```python
from build123d import *

# Parameters (mm, degrees)
SKETCH1_W                 = 20
SKETCH1_H                 = 101.6
BASE_FLANGE1_DEPTH        = 0.7366
EDGE_FLANGE1_DEPTH        = 40.191036667
EDGE_FLANGE1_START        = 0.7366
EDGE_FLANGE1_FLAT_DEPTH   = 0.7366
CUT_EXTRUDE1_DEPTH        = 235.985755194
CUT_EXTRUDE1_DEPTH_BACK   = 235.985755194
SKETCH9_R                 = 2
CUT_EXTRUDE3_DEPTH        = 238.044873218
CUT_EXTRUDE3_DEPTH_BACK   = 238.044873218
SKETCH11_R                = 3.96875
CUT_EXTRUDE5_DEPTH        = 196.726274862
CUT_EXTRUDE5_DEPTH_BACK   = 196.726274862
SKETCH13_R                = 1.984375
SKETCH13_R_2              = 1.190625
EDGE_FLANGE2_DEPTH        = 54.2634
EDGE_FLANGE2_START        = 0.7366
EDGE_FLANGE2_FLAT_DEPTH   = 0.7366
EDGE_FLANGE2_BEND_DEPTH   = 54.2634
EDGE_FLANGE2_FLAT_2_DEPTH = 0.7366
SKETCH30_R                = 9.089973339
CUT_EXTRUDE15_DEPTH       = 10


# Sheet-metal steps are written as plain solids
with BuildPart() as part:
    # Sketch1 → Base-Flange1 (new body)
    with BuildSketch(Plane(origin=(0, 0, 0), x_dir=(1, 0, 0), z_dir=(0, 1, 0))):
        Rectangle(SKETCH1_W, SKETCH1_H)
    extrude(amount=-BASE_FLANGE1_DEPTH)

    # Edge-Flange1 bend section (across the edge) → Edge-Flange1 (add)
    with BuildSketch(Plane(origin=(-11, 0, -15.686713846), x_dir=(1, 0, 0), z_dir=(0, 0, 1))):
        with BuildLine():
            Line((-0.7366, 0.7366), (0, 0.7366))
            ThreePointArc((0, 0.7366), (0.215745145, 0.215745145), (0.7366, 0))
            Line((0.7366, 0), (1, 0))
            Line((1, 0), (1, -0.7366))
            Line((1, -0.7366), (0.7366, -0.7366))
            ThreePointArc((0.7366, -0.7366), (-0.30510971, -0.30510971), (-0.7366, 0.7366))
        make_face()
    extrude(amount=EDGE_FLANGE1_DEPTH)

    # Edge-Flange1 profile (on flange) → Edge-Flange1 flat (add)
    with BuildSketch(Plane.ZY.offset(11).offset(EDGE_FLANGE1_START)):
        with BuildLine():
            ThreePointArc((24.504322822, 55), (4.408804488, 72.976240445), (-15.686713846, 55))
            Line((-15.686713846, 55), (-15.686713846, 0.7366))
            Line((-15.686713846, 0.7366), (24.504322822, 0.7366))
            Line((24.504322822, 0.7366), (24.504322822, 55))
        make_face()
    extrude(amount=-EDGE_FLANGE1_FLAT_DEPTH)

    # Sketch9 → Cut-Extrude1 (cut, two sides: drawn at the far end of the back side and taken through both)
    with BuildSketch(Plane(origin=(-32.365, -124.793980752, 68.826299478), x_dir=(0, 0, -1), z_dir=(1, 0, 0)).offset(-CUT_EXTRUDE1_DEPTH_BACK)):
        with Locations(Location((68.826299478, 136.507533033, 0), (0, 0, 270))):
            Circle(SKETCH9_R)
    extrude(amount=CUT_EXTRUDE1_DEPTH + CUT_EXTRUDE1_DEPTH_BACK, mode=Mode.SUBTRACT)

    # Sketch11 → Cut-Extrude3 (cut, two sides: drawn at the far end of the back side and taken through both)
    with BuildSketch(Plane(origin=(-42.6, -124.793980752, 68.826299478), x_dir=(0, 0, -1), z_dir=(1, 0, 0)).offset(-CUT_EXTRUDE3_DEPTH_BACK)):
        with Locations(Location((61.354566786, 177.878571708, 0), (0, 0, 270))):
            Circle(SKETCH11_R)
    extrude(amount=CUT_EXTRUDE3_DEPTH + CUT_EXTRUDE3_DEPTH_BACK, mode=Mode.SUBTRACT)

    # Sketch13 → Cut-Extrude5 (cut, two sides: drawn at the far end of the back side and taken through both)
    with BuildSketch(Plane(origin=(124.911822879, 0, 68.826299478), x_dir=(-0.7071067811865436, 0, 0.7071067811865515), z_dir=(0, 1, 0)).offset(-CUT_EXTRUDE5_DEPTH_BACK)):
        with Locations(Location((68.508410595, -102.424928038, 0), (0, 0, 45))):
            Circle(SKETCH13_R)
        with Locations(Location((68.508410595, -113.219195896, 0), (0, 0, 45))):
            Circle(SKETCH13_R_2)
        with Locations(Location((5.089841868, -165.843496765, 0), (0, 0, 45))):
            Circle(SKETCH13_R)
        with Locations(Location((15.884109726, -165.843496765, 0), (0, 0, 45))):
            Circle(SKETCH13_R_2)
    extrude(amount=CUT_EXTRUDE5_DEPTH + CUT_EXTRUDE5_DEPTH_BACK, mode=Mode.SUBTRACT)

    # Edge-Flange2 bend section (across the edge) → Edge-Flange2 (add)
    with BuildSketch(Plane(origin=(-11, 0.7366, -16.686713846), x_dir=(0, 0, 1), z_dir=(0, 1, 0))):
        with BuildLine():
            Line((-0.7366, 0.7366), (0, 0.7366))
            ThreePointArc((0, 0.7366), (0.215745145, 0.215745145), (0.7366, 0))
            Line((0.7366, 0), (1, 0))
            Line((1, 0), (1, -0.7366))
            Line((1, -0.7366), (0.7366, -0.7366))
            ThreePointArc((0.7366, -0.7366), (-0.30510971, -0.30510971), (-0.7366, 0.7366))
        make_face()
    extrude(amount=EDGE_FLANGE2_DEPTH)

    # Edge-Flange2 profile (on flange) → Edge-Flange2 flat (add)
    with BuildSketch(Plane(origin=(-11, 0, -16.686713846), x_dir=(0, 1, 0), z_dir=(0, 0, -1)).offset(EDGE_FLANGE2_START)):
        with BuildLine():
            Line((50, 9.2634), (0.7366, 9.2634))
            Line((0.7366, 9.2634), (0.7366, 0.7366))
            Line((0.7366, 0.7366), (55, 0.7366))
            Line((55, 0.7366), (55, 4.2634))
            ThreePointArc((55, 4.2634), (53.535533906, 7.798933906), (50, 9.2634))
        make_face()
    extrude(amount=-EDGE_FLANGE2_FLAT_DEPTH)

    # Edge-Flange2 bend section 2 (across the edge) → Edge-Flange2 bend (add)
    with BuildSketch(Plane(origin=(-11, 55, 25.504322822), x_dir=(0, 0, -1), z_dir=(0, -1, 0))):
        with BuildLine():
            Line((-0.7366, 0.7366), (0, 0.7366))
            ThreePointArc((0, 0.7366), (0.215745145, 0.215745145), (0.7366, 0))
            Line((0.7366, 0), (1, 0))
            Line((1, 0), (1, -0.7366))
            Line((1, -0.7366), (0.7366, -0.7366))
            ThreePointArc((0.7366, -0.7366), (-0.30510971, -0.30510971), (-0.7366, 0.7366))
        make_face()
    extrude(amount=EDGE_FLANGE2_BEND_DEPTH)

    # Edge-Flange2 profile 2 (on flange) → Edge-Flange2 flat 2 (add)
    with BuildSketch(Plane(origin=(-11, 0, 25.504322822), x_dir=(0, -1, 0), z_dir=(0, 0, 1)).offset(EDGE_FLANGE2_START)):
        with BuildLine():
            ThreePointArc((-50, 9.2634), (-53.535533906, 7.798933906), (-55, 4.2634))
            Line((-55, 4.2634), (-55, 0.7366))
            Line((-55, 0.7366), (-0.7366, 0.7366))
            Line((-0.7366, 0.7366), (-0.7366, 9.2634))
            Line((-0.7366, 9.2634), (-50, 9.2634))
        make_face()
    extrude(amount=-EDGE_FLANGE2_FLAT_2_DEPTH)

    # Sketch30 → Cut-Extrude15 (cut)
    with BuildSketch(Plane(origin=(-11, 0, 0), x_dir=(0, 0, -1), z_dir=(1, 0, 0))):
        with Locations(Location((-3.816431775, 31.863348386, 0), (0, 0, 90))):
            Circle(SKETCH30_R)
    extrude(amount=-CUT_EXTRUDE15_DEPTH, mode=Mode.SUBTRACT)


solid = part.part
```
Work out the finished part from the listing and answer in its coordinate system (mm). A direction names the side the tool comes from. Round coordinates to 2 decimals unless told otherwise and drop trailing zeros. Loops run counter-clockwise (first coordinate to the right, second up) from the corner with the lowest first, then second, coordinate; pieces in that order, holes last. Notation, with made-up numbers: (22.25, -29) -> (53.25, -29) arc R12 ccw to (53.25, -12) -> close; hole circle Ø5 at (-14.5, 63). An arc over 180 degrees is marked (long way). Write each question's results on one line, items separated by ' | '. Start each with the question number.
1. Section D-D (x = 7.25) is taken. Determine the outline of the cut face in (y, z).
2. A tool of negligible diameter and unlimited length cuts with its end or side. For faces 5 (the face through (-4.31, -0.37, -38.16)), 6 (the face through (-6, 28, 25.504)), 7 (the face through (-6, 27, -17.423)), from which of +Z, -Z, +X, -X, +Y, -Y can it reach the whole face along a straight path? Write none if from no direction.
3. Section A-A (z = 9) is taken. Determine the outline of the cut face in (x, y), plus the area to 3 significant figures.
4. Section B-B (y = 27) is taken. Determine the outline of the cut face in (x, z).
5. Section C-C (y = 44) is taken. Determine the outline of the cut face in (x, z), plus the area to 3 significant figures.
6. For a pull along Z with two mould halves and no side action, classify faces 1 (the face through (-11, 37, -4)), 2 (the face through (-3.162, 53.496, 25.878)), 3 (the face through (-6, 27, -16.687)), 4 (the face through (-6, 28, 26.241)) as +Z half, -Z half, draft (parallel to the pull), parting line (faces both ways), or undercut.
7. Find the intervals of material crossed by probe 1 along Z at (x, y) = (-8.75, 22.5); probe 2 along X at (y, z) = (43.5, -14); probe 3 along Y at (x, z) = (-6, 43.5), in increasing order. Write a range as from..to.
8. Given pin 1 Ø16.5 at (y, z) = (31.86, 3.82) entering from +X; pin 2 Ø2 at (x, y) = (-6.5, 27) entering from -Z; pin 3 Ø4.5 at (y, z) = (11.71, 0) entering from -X; pin 4 Ø0.8 at (y, z) = (-0.5, 33) entering from -X, each flat-ended and moving along its own axis, determine where each tip first touches the part or whether it passes through.
Evaluation:
1) outline: (-0.74, -50.8) -> (0, -50.8) -> (0, 50.8) -> (-0.74, 50.8) -> close
2) face 5: +Y, -Y | face 6: +X, +Y | face 7: -Z, +X, -X, +Y
3) outline: (-11.74, 0.74) arc R1.47 ccw to (-10.26, -0.74) -> (10, -0.74) -> (10, 0) -> (-10.26, 0) arc R0.74 cw to (-11, 0.74) -> (-11, 24.4) -> (-11.74, 24.4) -> close; (-11.74, 39.33) -> (-11, 39.33) -> (-11, 49.42) -> (-11.74, 49.42) -> close; (-11.74, 56.75) -> (-11, 56.75) -> (-11, 72.45) -> (-11.74, 72.45) -> close | area: 52.6 mm2
4) outline: (-11.74, -15.95) arc R1.47 ccw to (-10.26, -17.42) -> (-1.74, -17.42) -> (-1.74, -16.69) -> (-10.26, -16.69) arc R0.74 cw to (-11, -15.95) -> (-11, -3.86) -> (-11.74, -3.86) -> close; (-11.74, 11.5) -> (-11, 11.5) -> (-11, 24.77) arc R0.74 cw to (-10.26, 25.5) -> (-1.74, 25.5) -> (-1.74, 26.24) -> (-10.26, 26.24) arc R1.47 ccw to (-11.74, 24.77) -> close
5) outline: (-11.74, -15.95) arc R1.47 ccw to (-10.26, -17.42) -> (-1.74, -17.42) -> (-1.74, -16.69) -> (-10.26, -16.69) arc R0.74 cw to (-11, -15.95) -> (-11, 24.77) arc R0.74 cw to (-10.26, 25.5) -> (-1.74, 25.5) -> (-1.74, 26.24) -> (-10.26, 26.24) arc R1.47 ccw to (-11.74, 24.77) -> close | area: 45.1 mm2
6) face 1: undercut | face 2: draft | face 3: undercut | face 4: +Z half
7) probe 1: z = -17.42..-16.69, 25.5..26.24 | probe 2: x = -11.74..-11 | probe 3: y = -0.74..0
8) pin 1: passes through | pin 2: stops at z = -17.42 | pin 3: stops at x = -11.74 | pin 4: stops at x = -10
